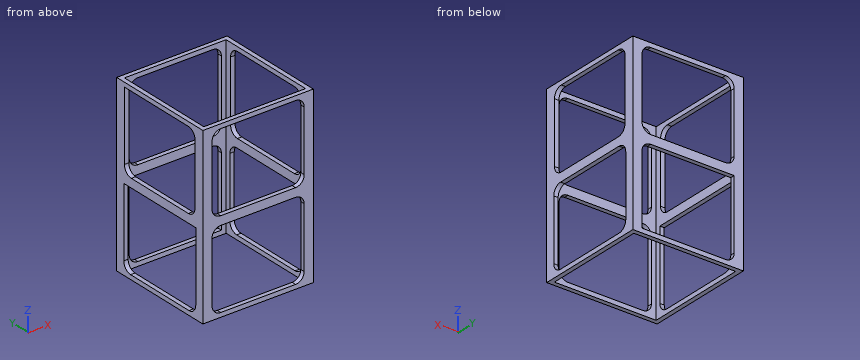
from build123d import *

# Parameters (mm, degrees)
F0_W     = 63.5
F0_H     = 63.5
F0_W_2   = 58.5
F0_H_2   = 58.5
F1_DEPTH = 100
F2_W     = 53
F2_H     = 45
F3_DEPTH = 63.501
F4_W     = 53
F4_H     = 45
F4_W_2   = 52
F5_DEPTH = 63.501
F6_R     = 5
F7_R     = 5


with BuildPart() as f1:
    # F0 (on Top) → F1 (new body)
    with BuildSketch(Plane.XY):
        Rectangle(F0_W, F0_H)
        Rectangle(F0_W_2, F0_H_2, mode=Mode.SUBTRACT)
    extrude(amount=F1_DEPTH)

    # F2 (on face) → F3 (cut, through all)
    with BuildSketch(Plane.XZ.offset(31.75)):
        with Locations((0, 75)):
            Rectangle(F2_W, F2_H)
        with Locations((0, 25)):
            Rectangle(F2_W, F2_H)
    extrude(amount=-F3_DEPTH, mode=Mode.SUBTRACT)

    # F4 (on face) → F5 (cut, through all)
    with BuildSketch(Plane(origin=(-31.75, 0, 0), x_dir=(0, -1, 0), z_dir=(-1, 0, 0))):
        with Locations((0, 25)):
            Rectangle(F4_W, F4_H)
        with Locations((0, 75)):
            Rectangle(F4_W_2, F4_H)
    extrude(amount=-F5_DEPTH, mode=Mode.SUBTRACT)

    # F6
    f6_edges = [f1.edges().sort_by_distance(p)[0] for p in [
        (30.5, -26.5, 2.5),
        (30.5, -26, 52.5),
        (-26.5, 30.5, 2.5),
        (-30.5, 26.5, 2.5),
        (-26.5, -30.5, 2.5),
        (-26.5, -30.5, 52.5),
        (-26.5, 30.5, 52.5),
        (-30.5, 26, 52.5),
        (30.5, 26, 52.5),
        (26.5, -30.5, 2.5),
        (26.5, -30.5, 52.5),
        (26.5, 30.5, 52.5),
        (-30.5, -26.5, 2.5),
        (-30.5, -26, 52.5),
    ]]
    fillet(f6_edges, radius=F6_R)

    # F7
    f7_edges = [f1.edges().sort_by_distance(p)[0] for p in [
        (30.5, 26, 97.5),
        (30.5, 26.5, 47.5),
        (-26.5, -30.5, 47.5),
        (-26.5, -30.5, 97.5),
        (30.5, 26.5, 2.5),
        (-26.5, 30.5, 97.5),
        (26.5, 30.5, 97.5),
        (30.5, -26, 97.5),
        (26.5, -30.5, 97.5),
        (30.5, -26.5, 47.5),
        (26.5, -30.5, 47.5),
        (26.5, 30.5, 47.5),
        (-30.5, -26, 97.5),
    ]]
    fillet(f7_edges, radius=F7_R)


solid = f1.part
For this review, take the finished solid that the model builds, in its own axes (mm). Give positions to 0.01 mm unless a question says otherwise; leave off trailing zeros. Order: outer loops, then holes, each group sorted by start corner. A loop starts at its lowest first (then second) coordinate and runs counter-clockwise, first axis right, second up. Notation, with made-up numbers: (77, 4.5) - (114, 4.5) arc R12 ccw to (114, 15.5) - close; hole circle Ø10 at (51.5, 79.25). An arc over 180 degrees is marked (long way). Answer as a JSON object with one key per item and string values. Group by question number.
Item 1: Take a section at A-A on y = 11. Give the boundary of the cut face in (x, z).
Item 2: Wall thickness on line 1 along X through (y, z) = (-27, 60.5); line 2 along X through (y, z) = (29.5, 73): over which ranges is each line inside the solid? List them lowest first.
Item 3: Take a section at C-C on z = 88. Give the boundary of the cut face in (x, y).
Item 4: Take a section at D-D on z = 28.5. Give the boundary of the cut face in (x, y), and give its area (3 significant figures).
Reported:
{
 "1": {"outline": "(-31.75, 0) - (-29.25, 0) - (-29.25, 2.5) - (-31.75, 2.5) - close; (-31.75, 47.5) - (-29.25, 47.5) - (-29.25, 52.5) - (-31.75, 52.5) - close; (-31.75, 97.5) - (-29.25, 97.5) - (-29.25, 100) - (-31.75, 100) - close; (29.25, 0) - (31.75, 0) - (31.75, 2.5) - (29.25, 2.5) - close; (29.25, 47.5) - (31.75, 47.5) - (31.75, 52.5) - (29.25, 52.5) - close; (29.25, 97.5) - (31.75, 97.5) - (31.75, 100) - (29.25, 100) - close"},
 "2": {"line 1": "-31.75 to -29.25, 29.25 to 31.75", "line 2": "-31.75 to -26.5, 26.5 to 31.75"},
 "3": {"outline": "(-31.75, -31.75) - (-26.5, -31.75) - (-26.5, -29.25) - (-29.25, -29.25) - (-29.25, -26) - (-31.75, -26) - close; (-31.75, 26) - (-29.25, 26) - (-29.25, 29.25) - (-26.5, 29.25) - (-26.5, 31.75) - (-31.75, 31.75) - close; (26.5, -31.75) - (31.75, -31.75) - (31.75, -26) - (29.25, -26) - (29.25, -29.25) - (26.5, -29.25) - close; (26.5, 29.25) - (29.25, 29.25) - (29.25, 26) - (31.75, 26) - (31.75, 31.75) - (26.5, 31.75) - close"},
 "4": {"outline": "(-31.75, -31.75) - (-26.5, -31.75) - (-26.5, -29.25) - (-29.25, -29.25) - (-29.25, -26.5) - (-31.75, -26.5) - close; (-31.75, 26.5) - (-29.25, 26.5) - (-29.25, 29.25) - (-26.5, 29.25) - (-26.5, 31.75) - (-31.75, 31.75) - close; (26.5, -31.75) - (31.75, -31.75) - (31.75, -26.5) - (29.25, -26.5) - (29.25, -29.25) - (26.5, -29.25) - close; (26.5, 29.25) - (29.25, 29.25) - (29.25, 26.5) - (31.75, 26.5) - (31.75, 31.75) - (26.5, 31.75) - close", "area": "80.0 mm^2"}
}
